Here's how the part is built. I have some questions about the finished solid (model axes, mm). Face numbers are marked on the shaded views. Coordinates: 2 decimals unless noted, no trailing zeros. Order: outer loops, then holes, each group sorted by start corner. A loop starts at its lowest first (then second) coordinate and runs counter-clockwise, first axis right, second up. Notation, with made-up numbers: (53, 19) - (105, 19) arc R12 ccw to (105, 39) - close; hole circle Ø3 at (68, -18). An arc over 180 degrees is marked (long way). Answer in a Markdown table with one row per item. Add a question column.
Item 1: I want a section at B-B (z = -2.5). Please give me the cut outline in (x, y), plus the area to 3 significant figures.
Item 2: If I drill on line 1 along Y through (x, z) = (-0.25, -2.7); line 2 along Y through (x, z) = (2, -2.4); line 3 along X through (y, z) = (-3, -1.55), over which ranges is the centre line in solid material (lowest first)? Write a range as from..to.
Item 3: Thinking about a two-plate mould opening in X: for the marked faces 1, 2, 3 and 4, which applies, +X half, -X half, draft (parallel to the pull), parting line (faces both ways), or undercut?
Item 4: I want a section at A-A (x = -0.25). Please give me the cut outline in (y, z).
Item 5: Will these pins go through, and if not, where does the flat tip stop? pin 1 Ø2 at (x, z) = (-2.5, -1.5) entering from -Y; pin 2 Ø1.3 at (x, y) = (0, -7) entering from -Z; pin 3 Ø2 at (x, z) = (7.5, -3) entering from -Y.
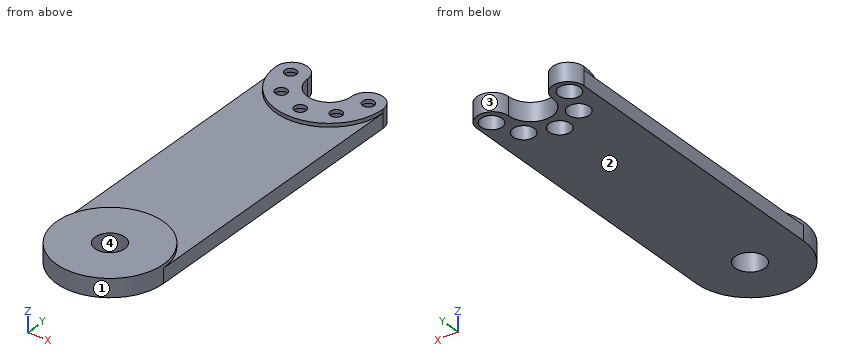
```python
from build123d import *

# Parameters (mm, degrees)
RESSALTO_EXTRUS_O1_DEPTH          = 0.75
RESSALTO_EXTRUS_O2_DEPTH          = 3
REBAIXO_PARA_SHCS_M21_D           = 2.4
REBAIXO_PARA_SHCS_M21_CBORE_D     = 4.4
REBAIXO_PARA_SHCS_M21_CBORE_DEPTH = 3
RESSALTO_EXTRUS_O3_START          = 0.75
ESBO_O4_R                         = 11
RESSALTO_EXTRUS_O3_DEPTH          = 0.75
ESBO_O5_R                         = 3.05
CORTE_EXTRUS_O1_DEPTH             = 72.944857356


with BuildPart() as part:
    # Esboço1 → Ressalto-extrusão1 (new body)
    with BuildSketch(Plane.XY):
        with BuildLine():
            ThreePointArc((-4.5, 0), (0, -4.5), (4.5, 0))
            ThreePointArc((4.5, 0), (7.75, 3.25), (11, 0))
            ThreePointArc((11, 0), (0, -11), (-11, 0))
            ThreePointArc((-11, 0), (-7.75, 3.25), (-4.5, 0))
        make_face()
    extrude(amount=-RESSALTO_EXTRUS_O1_DEPTH)

    # Esboço3 → Ressalto-extrusão2 (add)
    with BuildSketch(Plane(origin=(0, 0, -0.75), x_dir=(-1, 0, 0), z_dir=(0, 0, -1))):
        with BuildLine():
            Line((-11, 0), (-11, -60))
            ThreePointArc((-11, -60), (0, -71), (11, -60))
            Line((11, -60), (11, 0))
            ThreePointArc((11, 0), (7.75, 3.25), (4.5, 0))
            ThreePointArc((4.5, 0), (0, -4.5), (-4.5, 0))
            ThreePointArc((-4.5, 0), (-7.75, 3.25), (-11, 0))
        make_face()
    extrude(amount=RESSALTO_EXTRUS_O2_DEPTH)

    # Rebaixo para SHCS M21 (through all)
    with Locations(Plane(origin=(0, 0, -3.75), x_dir=(-1, 0, 0), z_dir=(0, 0, -1))):
        with Locations((-8, 0), (-5.656854249, -5.656854249), (0, -8), (5.656854249, -5.656854249), (8, 0)):
            CounterBoreHole(REBAIXO_PARA_SHCS_M21_D / 2, REBAIXO_PARA_SHCS_M21_CBORE_D / 2, REBAIXO_PARA_SHCS_M21_CBORE_DEPTH)

    # Esboço4 → Ressalto-extrusão3 (add)
    with BuildSketch(Plane.XY.offset(-0.75).offset(RESSALTO_EXTRUS_O3_START)):
        with Locations((0, -60)):
            Circle(ESBO_O4_R)
    extrude(amount=-RESSALTO_EXTRUS_O3_DEPTH)

    # Esboço5 → Corte-extrusão1 (cut, through all)
    with BuildSketch(Plane(origin=(0, 0, -3.75), x_dir=(-1, 0, 0), z_dir=(0, 0, -1))):
        with Locations((0, -60)):
            Circle(ESBO_O5_R)
    extrude(amount=-CORTE_EXTRUS_O1_DEPTH, mode=Mode.SUBTRACT)


solid = part.part
```
Values follow:
| question | item | result |
|---|---|---|
| 1 | outline | (-11, -60) arc R11 ccw to (11, -60) - (11, 0) arc R3.25 ccw to (4.5, 0) arc R4.5 cw to (-4.5, 0) arc R3.25 ccw to (-11, 0) - close; hole circle Ø4.4 at (-8, 0); hole circle Ø4.4 at (-5.66, -5.66); hole circle Ø6.1 at (0, -60); hole circle Ø4.4 at (0, -8); hole circle Ø4.4 at (5.66, -5.66); hole circle Ø4.4 at (8, 0) |
| 1 | area | 1,410 mm^2 |
| 2 | line 1 | y = -71..-63.04, -56.96..-10.19, -5.81..-4.49 |
| 2 | line 2 | y = -70.82..-62.3, -57.7..-8.92, -7.08..-4.03 |
| 2 | line 3 | x = -11..-3.35, 3.35..11 |
| 3 | face 1 | parting line |
| 3 | face 2 | draft |
| 3 | face 3 | undercut |
| 3 | face 4 | undercut |
| 4 | outline | (-71, -3.75) - (-63.04, -3.75) - (-63.04, 0) - (-71, 0) - close; (-56.96, -3.75) - (-10.19, -3.75) - (-10.19, -0.75) - (-9.17, -0.75) - (-9.17, 0) - (-11, 0) - (-11, -0.75) - (-49, -0.75) - (-49, 0) - (-56.96, 0) - close; (-6.83, -0.75) - (-5.81, -0.75) - (-5.81, -3.75) - (-4.49, -3.75) - (-4.49, 0) - (-6.83, 0) - close |
| 5 | pin 1 | stops at y = -70.9 |
| 5 | pin 2 | stops at z = -0.75 |
| 5 | pin 3 | stops at y = -68.87 |
